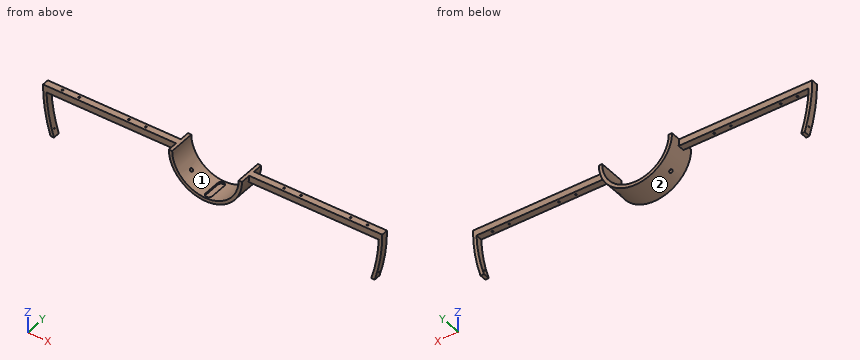
```python
from build123d import *

# Parameters (mm, degrees)
BOSS_EXTRUDE1_DEPTH = 80
SKETCH2_W           = 20
SKETCH2_H           = 10
BOSS_EXTRUDE2_DEPTH = 400
SKETCH3_W           = 20
SKETCH3_H           = 20
BOSS_EXTRUDE3_DEPTH = 400
BOSS_EXTRUDE4_DEPTH = 20
BOSS_EXTRUDE5_DEPTH = 20
SKETCH10_R          = 2.5
CUT_EXTRUDE1_DEPTH  = 20
SKETCH11_R          = 5
CUT_EXTRUDE3_DEPTH  = 20
SKETCH12_R          = 5
CUT_EXTRUDE4_DEPTH  = 20
SKETCH15_W          = 10
SKETCH15_H          = 50
CUT_EXTRUDE7_DEPTH  = 15
SKETCH16_R          = 1.5
CUT_EXTRUDE8_DEPTH  = 50
SKETCH17_R          = 1.5
CUT_EXTRUDE9_DEPTH  = 50


with BuildPart() as part:
    # Sketch1 → Boss-Extrude1 (new body)
    with BuildSketch(Plane(origin=(0, 0, 0), x_dir=(1, 0, 0), z_dir=(0, 1, 0))):
        with BuildLine():
            Line((-110, 0), (-100, 0))
            ThreePointArc((-100, 0), (0, 100), (100, 0))
            Line((100, 0), (110, 0))
            ThreePointArc((110, 0), (0, 110), (-110, 0))
        make_face()
    extrude(amount=BOSS_EXTRUDE1_DEPTH)

    # Sketch2 → Boss-Extrude2 (add)
    with BuildSketch(Plane(origin=(100, 80, 0), x_dir=(0, 0, 1), z_dir=(-1, 0, 0))):
        with Locations((-10, -35)):
            Rectangle(SKETCH2_W, SKETCH2_H)
        with Locations((-10, -45)):
            Rectangle(SKETCH2_W, SKETCH2_H)
    extrude(amount=-BOSS_EXTRUDE2_DEPTH)

    # Sketch3 → Boss-Extrude3 (add)
    with BuildSketch(Plane(origin=(-100, 80, 0), x_dir=(0, 0, -1), z_dir=(1, 0, 0))):
        with Locations((10, -40)):
            Rectangle(SKETCH3_W, SKETCH3_H)
    extrude(amount=-BOSS_EXTRUDE3_DEPTH)

    # Sketch5 → Boss-Extrude4 (add)
    with BuildSketch(Plane(origin=(0, 50, 0), x_dir=(1, 0, 0), z_dir=(0, 1, 0))):
        with BuildLine():
            Line((500, 0), (510, 0))
            ThreePointArc((510, 0), (504.329046943, 75.843341231), (487.442304278, 150))
            Line((487.442304278, 150), (476.969600708, 150))
            ThreePointArc((476.969600708, 150), (494.208862908, 75.878849641), (500, 0))
        make_face()
    extrude(amount=-BOSS_EXTRUDE4_DEPTH)

    # Sketch7 → Boss-Extrude5 (add)
    with BuildSketch(Plane(origin=(0, 50, 0), x_dir=(1, 0, 0), z_dir=(0, 1, 0))):
        with BuildLine():
            ThreePointArc((-510, 0), (-504.329046943, 75.843341231), (-487.442304278, 150))
            Line((-487.442304278, 150), (-476.969600708, 150))
            ThreePointArc((-476.969600708, 150), (-494.208862908, 75.878849641), (-500, 0))
            Line((-500, 0), (-510, 0))
        make_face()
    extrude(amount=-BOSS_EXTRUDE5_DEPTH)

    # Sketch10 → Cut-Extrude1 (cut)
    with BuildSketch(Plane(origin=(0, 0, -20), x_dir=(-1, 0, 0), z_dir=(0, 0, -1))):
        with Locations((-258.166538264, 40)):
            Circle(SKETCH10_R)
        with Locations((-408.166538264, 40)):
            Circle(SKETCH10_R)
        with Locations((258.166538264, 40)):
            Circle(SKETCH10_R)
        with Locations((408.166538264, 40)):
            Circle(SKETCH10_R)
        with Locations((-458.166538264, 40)):
            Circle(SKETCH10_R)
        with Locations((-208.166538264, 40)):
            Circle(SKETCH10_R)
        with Locations((208.166538264, 40)):
            Circle(SKETCH10_R)
        with Locations((458.166538264, 40)):
            Circle(SKETCH10_R)
    extrude(amount=-CUT_EXTRUDE1_DEPTH, mode=Mode.SUBTRACT)

    # Sketch11 → Cut-Extrude3 (cut)
    with BuildSketch(Plane(origin=(-77.781745931, 0, -77.781745931), x_dir=(-0.707106781, 0, 0.707106781), z_dir=(-0.707106781, 0, -0.707106781))):
        with Locations((0, 40)):
            Circle(SKETCH11_R)
    extrude(amount=-CUT_EXTRUDE3_DEPTH, mode=Mode.SUBTRACT)

    # Sketch12 → Cut-Extrude4 (cut)
    with BuildSketch(Plane(origin=(77.781745931, 0, -77.781745931), x_dir=(-0.707106781, 0, -0.707106781), z_dir=(0.707106781, 0, -0.707106781))):
        with Locations((0, 40)):
            Circle(SKETCH12_R)
    extrude(amount=-CUT_EXTRUDE4_DEPTH, mode=Mode.SUBTRACT)

    # Sketch15 → Cut-Extrude7 (cut)
    with BuildSketch(Plane.XY.offset(-90)):
        with BuildLine():
            ThreePointArc((-10, 15), (-7.071067812, 7.928932188), (0, 5))
            Line((0, 5), (0, 15))
            Line((0, 15), (-10, 15))
        make_face()
        with BuildLine():
            Line((0, 15), (0, 5))
            ThreePointArc((0, 5), (7.071067812, 7.928932188), (10, 15))
            Line((10, 15), (0, 15))
        make_face()
        with Locations((5, 40)):
            Rectangle(SKETCH15_W, SKETCH15_H)
        with Locations((-5, 40)):
            Rectangle(SKETCH15_W, SKETCH15_H)
        with BuildLine():
            Line((-10, 65), (0, 65))
            Line((0, 65), (0, 75))
            ThreePointArc((0, 75), (-7.071067812, 72.071067812), (-10, 65))
        make_face()
        with BuildLine():
            Line((0, 75), (0, 65))
            Line((0, 65), (10, 65))
            ThreePointArc((10, 65), (7.071067812, 72.071067812), (0, 75))
        make_face()
    extrude(amount=-CUT_EXTRUDE7_DEPTH, mode=Mode.SUBTRACT)

    # Sketch16 → Cut-Extrude8 (cut)
    with BuildSketch(Plane(origin=(-510, 30, 0), x_dir=(0, 0, 1), z_dir=(-1, 0, 0))):
        with Locations((-130, 10)):
            Circle(SKETCH16_R)
    extrude(amount=-CUT_EXTRUDE8_DEPTH, mode=Mode.SUBTRACT)

    # Sketch17 → Cut-Extrude9 (cut)
    with BuildSketch(Plane(origin=(510, 30, 0), x_dir=(0, 0, -1), z_dir=(1, 0, 0))):
        with Locations((130, 10)):
            Circle(SKETCH17_R)
    extrude(amount=-CUT_EXTRUDE9_DEPTH, mode=Mode.SUBTRACT)


solid = part.part
```
Geometry: final body of the model. Coordinates: model frame, mm. Face numbers are marked on the shaded views. Round coordinates to 2 decimals unless told otherwise and drop trailing zeros. Order: outer loops, then holes, each group sorted by start corner. A loop starts at its lowest first (then second) coordinate and runs counter-clockwise, first axis right, second up. Notation, with made-up numbers: (84.25, -5) -> (104.25, -5) arc R22 cw to (104.25, 16) -> close; hole circle Ø1 at (46, -4). An arc over 180 degrees is marked (long way). Use one line per item in the form item = value.
(1) Section A-A on x = 303.5. Return loops of the section in (y, z).
Results list:
outline = (30, -20) -> (50, -20) -> (50, 0) -> (30, 0) -> close
(2) Draft query along X for the marked faces 1 and 2. Return one class per face: pulls with the +X half, pulls with the -X half, needs draft (parallel to the pull), parting line crosses it, or undercut.
Results list:
face_1 = undercut
face_2 = undercut
(3) Ray query, probe 1 along X at (y, z) = (47.5, -79); probe 2 along X at (y, z) = (35.5, -30.5); probe 3 along Y at (x, z) = (490.75, -130). Return the intervals inside material, ascending. Write a range as [from, to].
Results list:
probe_1 = [-503.84, -493.72], [-76.54, -61.31], [61.31, 76.54], [493.72, 503.84]
probe_2 = [-509.09, -499.07], [-105.69, -95.24], [95.24, 105.69], [499.07, 509.09]
probe_3 = [30, 38.5], [41.5, 50]
(4) First-contact query: pin 1 Ø6 at (x, y) = (458.17, 40) entering from -Z; pin 2 Ø2 at (y, z) = (28.5, -100.5) entering from +X; pin 3 Ø4 at (y, z) = (36.5, -47) entering from -X. Flat tips, straight axial feed; report the tip coordinate or a pass-through.
Results list:
pin_1 = -20
pin_2 = 46.9
pin_3 = -508.01
